For this review, take the finished solid that the model builds, in its own axes (mm). A direction names the side the tool comes from. Coordinates: 2 decimals unless noted, no trailing zeros. Loops run counter-clockwise (first coordinate to the right, second up) from the corner with the lowest first, then second, coordinate; pieces in that order, holes last. Notation, with made-up numbers: (33, -7) - (82, -7) arc R26 cw to (82, 21) - close; hole circle Ø5 at (81.25, 83). An arc over 180 degrees is marked (long way). One line per item, written item: value. Start each with the question number.
1. Take a section at C-C, the plane y = 12. State the section outline as (x, z) points.
2. Insertion check: pin 1 (6.5 mm diameter, centred on x = 22.5, z = -70.5, fed in from -Y); pin 2 (3 mm diameter, centred on x = -4, z = -31, fed in from -Y) (3 decimals). Each pin has a flat end and moves straight along its axis. Give the tip position at first contact, or say it passes through.
3. To check wall thickness, follow line 1 (Z direction, x = -4.5, y = 4); line 2 (X direction, y = 4.5, z = -4); line 3 (Z direction, x = 1, y = 3). State the ranges of each line that lie inside material, in increasing order. Write a range as from..to.
4. The part is to be moulded in two halves that separate along X. For faces 6 (the face through (0, 19.05, -1)), 7 (the face through (31.75, 9, 1)), 8 (the face through (0, 9, -76.2)), say which applies: released by +X, released by -X, zero draft, split by the parting line, or undercut.
5. For faces 1 (the face through (-28, 0, -16)), 2 (the face through (-0.1, 4.76, -89.08)), 3 (the face through (-25.078, 4.696, 95.027)), 4 (the face through (19.05, 14, -72)), 5 (the face through (-31.75, 9, 1)), list the 3-axis set-ups (+Z, -Z, +X, -X, +Y, -Y) from which the entire face can be reached by the end or side of a thin tool; tool diameter is ignored.
6. Take a section at D-D, the plane z = -48. State the section outline as (x, y) points, and give its area (3 significant figures).
```python
from build123d import *

# Parameters (mm, degrees)
SKETCH1_W           = 63.5
SKETCH1_H           = 203.2
BOSS_EXTRUDE1_DEPTH = 19.05
SKETCH2_R           = 4.7625
CUT_EXTRUDE1_DEPTH  = 25.4
CUT_EXTRUDE2_DEPTH  = 9.525
SKETCH5_W           = 38.1
SKETCH5_H           = 8.128
CUT_EXTRUDE4_DEPTH  = 109.136603424
SKETCH6_W           = 53.975
SKETCH6_H           = 33.655
CUT_EXTRUDE5_DEPTH  = 2.159


with BuildPart() as part:
    # Sketch1 → Boss-Extrude1 (new body)
    with BuildSketch(Plane(origin=(0, 0, 0), x_dir=(1, 0, 0), z_dir=(0, 1, 0))):
        Rectangle(SKETCH1_W, SKETCH1_H)
    extrude(amount=BOSS_EXTRUDE1_DEPTH)

    # Sketch2 → Cut-Extrude1 (cut)
    with BuildSketch(Plane(origin=(0, 0, -101.6), x_dir=(-1, 0, 0), z_dir=(0, 0, -1))):
        Circle(SKETCH2_R)
    extrude(amount=-CUT_EXTRUDE1_DEPTH, mode=Mode.SUBTRACT)

    # Sketch3 → Cut-Extrude2 (cut)
    with BuildSketch(Plane(origin=(0, 0, 0), x_dir=(-1, 0, 0), z_dir=(0, -1, 0))):
        with BuildLine():
            Line((-20.6375, -96.8375), (20.6375, -96.8375))
            ThreePointArc((20.6375, -96.8375), (25.127628061, -94.977628061), (26.9875, -90.4875))
            Line((26.9875, -90.4875), (26.9875, 37.592))
            ThreePointArc((26.9875, 37.592), (25.127628061, 42.082128061), (20.6375, 43.942))
            Line((20.6375, 43.942), (-20.6375, 43.942))
            ThreePointArc((-20.6375, 43.942), (-25.127628061, 42.082128061), (-26.9875, 37.592))
            Line((-26.9875, 37.592), (-26.9875, -90.4875))
            ThreePointArc((-26.9875, -90.4875), (-25.127628061, -94.977628061), (-20.6375, -96.8375))
        make_face()
        with BuildLine():
            Line((-23.8125, 76.2), (23.8125, 76.2))
            ThreePointArc((23.8125, 76.2), (26.05756403, 75.27006403), (26.9875, 73.025))
            Line((26.9875, 73.025), (26.9875, 71.247))
            ThreePointArc((26.9875, 71.247), (26.05756403, 69.00193597), (23.8125, 68.072))
            Line((23.8125, 68.072), (-23.8125, 68.072))
            ThreePointArc((-23.8125, 68.072), (-26.05756403, 69.00193597), (-26.9875, 71.247))
            Line((-26.9875, 71.247), (-26.9875, 73.025))
            ThreePointArc((-26.9875, 73.025), (-26.05756403, 75.27006403), (-23.8125, 76.2))
        make_face()
    extrude(amount=-CUT_EXTRUDE2_DEPTH, mode=Mode.SUBTRACT)

    # Sketch5 → Cut-Extrude4 (cut, through all)
    with BuildSketch(Plane(origin=(0, 0, 0), x_dir=(1, 0, 0), z_dir=(0, 1, 0))):
        with Locations((0, 72.136)):
            Rectangle(SKETCH5_W, SKETCH5_H)
    extrude(amount=CUT_EXTRUDE4_DEPTH, mode=Mode.SUBTRACT)

    # Sketch6 → Cut-Extrude5 (cut)
    with BuildSketch(Plane(origin=(0, 0, 0), x_dir=(1, 0, 0), z_dir=(0, 1, 0))):
        with Locations((0, 54.4195)):
            Rectangle(SKETCH6_W, SKETCH6_H)
    extrude(amount=CUT_EXTRUDE5_DEPTH, mode=Mode.SUBTRACT)


solid = part.part
```
Solutions:
1. outline: (-31.75, -101.6) - (31.75, -101.6) - (31.75, 101.6) - (-31.75, 101.6) - close; hole (-19.05, -76.2) - (19.05, -76.2) - (19.05, -68.07) - (-19.05, -68.07) - close
2. pin 1: y = 2.16
2. pin 2: y = 9.525
3. line 1: -101.6..-76.2, -68.07..-43.94, 96.84..101.6
3. line 2: -31.75..-26.99, 26.99..31.75
3. line 3: -68.07..-43.94, 96.84..101.6
4. face 6: zero draft
4. face 7: released by +X
4. face 8: undercut
5. face 1: +Z, -Z, +X, -X, -Y
5. face 2: -Z, -Y
5. face 3: -Y
5. face 4: +Y, -Y
5. face 5: +Z, -Z, -X, +Y, -Y
6. outline: (-31.75, 0) - (-26.99, 0) - (-26.99, 2.16) - (26.99, 2.16) - (26.99, 0) - (31.75, 0) - (31.75, 19.05) - (-31.75, 19.05) - close
6. area: 1,090 mm2
